from build123d import *

# Parameters (mm, degrees)
F1_DEPTH = 50.8
F2_DEPTH = 50.8
F3_DEPTH = 25.4
F4_DEPTH = 101.6
F5_SIZE  = 5
F6_R     = 5


with BuildPart() as f1:
    # F0 (on Front) → F1 (new body)
    with BuildSketch(Plane.XZ):
        with BuildLine():
            Line((-81.5396818683, 48.140194267), (-192.2345156552, 48.140194267))
            Line((-192.2345156552, 48.140194267), (-192.2345156552, 26.0968099283))
            ThreePointArc((-192.2345156552, 26.0968099283), (-174.3603015656, 18.6930680356), (-166.956559673, 0.8188539461))
            ThreePointArc((-166.956559673, 0.8188539461), (-174.3603015656, -17.0553601435), (-192.2345156552, -24.4591020361))
            Line((-192.2345156552, -24.4591020361), (-192.2345156552, -46.5024863749))
            Line((-192.2345156552, -46.5024863749), (-81.5396818683, -46.5024863749))
            ThreePointArc((-81.5396818683, -46.5024863749), (37.4445138693, -12.4899673839), (156.4287096069, -46.5024863749))
            Line((156.4287096069, -46.5024863749), (250.5448194923, -46.5024863749))
            Line((250.5448194923, -46.5024863749), (250.5448194923, -24.5132009882))
            ThreePointArc((250.5448194923, -24.5132009882), (225.212764558, 0.8188539461), (250.5448194923, 26.1509088804))
            Line((250.5448194923, 26.1509088804), (250.5448194923, 48.140194267))
            Line((250.5448194923, 48.140194267), (156.4287096069, 48.140194267))
            ThreePointArc((156.4287096069, 48.140194267), (37.4445138693, 1.7154132922), (-81.5396818683, 48.140194267))
        make_face()
    extrude(amount=F1_DEPTH)

    # F0 (on Front) → F2 (join)
    with BuildSketch(Plane.XZ):
        with BuildLine():
            Line((-81.5396818683, 48.140194267), (-192.2345156552, 48.140194267))
            Line((-192.2345156552, 48.140194267), (-192.2345156552, 26.0968099283))
            ThreePointArc((-192.2345156552, 26.0968099283), (-174.3603015656, 18.6930680356), (-166.956559673, 0.8188539461))
            ThreePointArc((-166.956559673, 0.8188539461), (-174.3603015656, -17.0553601435), (-192.2345156552, -24.4591020361))
            Line((-192.2345156552, -24.4591020361), (-192.2345156552, -46.5024863749))
            Line((-192.2345156552, -46.5024863749), (-81.5396818683, -46.5024863749))
            ThreePointArc((-81.5396818683, -46.5024863749), (37.4445138693, -12.4899673839), (156.4287096069, -46.5024863749))
            Line((156.4287096069, -46.5024863749), (250.5448194923, -46.5024863749))
            Line((250.5448194923, -46.5024863749), (250.5448194923, -24.5132009882))
            ThreePointArc((250.5448194923, -24.5132009882), (225.212764558, 0.8188539461), (250.5448194923, 26.1509088804))
            Line((250.5448194923, 26.1509088804), (250.5448194923, 48.140194267))
            Line((250.5448194923, 48.140194267), (156.4287096069, 48.140194267))
            ThreePointArc((156.4287096069, 48.140194267), (37.4445138693, 1.7154132922), (-81.5396818683, 48.140194267))
        make_face()
        with BuildLine():
            ThreePointArc((-166.956559673, 0.8188539461), (-174.3603015656, 18.6930680356), (-192.2345156552, 26.0968099283))
            Line((-192.2345156552, 26.0968099283), (-192.2345156552, 13.5188539461))
            ThreePointArc((-192.2345156552, 13.5188539461), (-183.2542595341, 9.7991100672), (-179.5345156552, 0.8188539461))
            ThreePointArc((-179.5345156552, 0.8188539461), (-183.2542595341, -8.161402175), (-192.2345156552, -11.8811460539))
            Line((-192.2345156552, -11.8811460539), (-192.2345156552, -24.4591020361))
            ThreePointArc((-192.2345156552, -24.4591020361), (-174.3603015656, -17.0553601435), (-166.956559673, 0.8188539461))
        make_face()
        with BuildLine():
            Line((-192.2345156552, 13.5188539461), (-192.2345156552, 26.0968099283))
            ThreePointArc((-192.2345156552, 26.0968099283), (-217.5124716374, 0.8188539461), (-192.2345156552, -24.4591020361))
            Line((-192.2345156552, -24.4591020361), (-192.2345156552, -11.8811460539))
            ThreePointArc((-192.2345156552, -11.8811460539), (-204.9345156552, 0.8188539461), (-192.2345156552, 13.5188539461))
        make_face()
        with BuildLine():
            ThreePointArc((275.8768744265, 0.8188539461), (268.4572873177, 18.7313217715), (250.5448194923, 26.1509088804))
            Line((250.5448194923, 26.1509088804), (250.5448194923, 13.5188539461))
            ThreePointArc((250.5448194923, 13.5188539461), (259.5250756133, 9.7991100672), (263.2448194923, 0.8188539461))
            ThreePointArc((263.2448194923, 0.8188539461), (259.5250756133, -8.161402175), (250.5448194923, -11.8811460539))
            Line((250.5448194923, -11.8811460539), (250.5448194923, -24.5132009882))
            ThreePointArc((250.5448194923, -24.5132009882), (268.4572873177, -17.0936138793), (275.8768744265, 0.8188539461))
        make_face()
        with BuildLine():
            Line((250.5448194923, 13.5188539461), (250.5448194923, 26.1509088804))
            ThreePointArc((250.5448194923, 26.1509088804), (225.212764558, 0.8188539461), (250.5448194923, -24.5132009882))
            Line((250.5448194923, -24.5132009882), (250.5448194923, -11.8811460539))
            ThreePointArc((250.5448194923, -11.8811460539), (237.8448194923, 0.8188539461), (250.5448194923, 13.5188539461))
        make_face()
    extrude(amount=F2_DEPTH)

    # F0 (on Front) → F3 (join)
    with BuildSketch(Plane.XZ):
        with BuildLine():
            Line((-81.5396818683, 48.140194267), (-192.2345156552, 48.140194267))
            Line((-192.2345156552, 48.140194267), (-192.2345156552, 26.0968099283))
            ThreePointArc((-192.2345156552, 26.0968099283), (-174.3603015656, 18.6930680356), (-166.956559673, 0.8188539461))
            ThreePointArc((-166.956559673, 0.8188539461), (-174.3603015656, -17.0553601435), (-192.2345156552, -24.4591020361))
            Line((-192.2345156552, -24.4591020361), (-192.2345156552, -46.5024863749))
            Line((-192.2345156552, -46.5024863749), (-81.5396818683, -46.5024863749))
            ThreePointArc((-81.5396818683, -46.5024863749), (37.4445138693, -12.4899673839), (156.4287096069, -46.5024863749))
            Line((156.4287096069, -46.5024863749), (250.5448194923, -46.5024863749))
            Line((250.5448194923, -46.5024863749), (250.5448194923, -24.5132009882))
            ThreePointArc((250.5448194923, -24.5132009882), (225.212764558, 0.8188539461), (250.5448194923, 26.1509088804))
            Line((250.5448194923, 26.1509088804), (250.5448194923, 48.140194267))
            Line((250.5448194923, 48.140194267), (156.4287096069, 48.140194267))
            ThreePointArc((156.4287096069, 48.140194267), (37.4445138693, 1.7154132922), (-81.5396818683, 48.140194267))
        make_face()
        with BuildLine():
            ThreePointArc((-166.956559673, 0.8188539461), (-174.3603015656, 18.6930680356), (-192.2345156552, 26.0968099283))
            Line((-192.2345156552, 26.0968099283), (-192.2345156552, 13.5188539461))
            ThreePointArc((-192.2345156552, 13.5188539461), (-183.2542595341, 9.7991100672), (-179.5345156552, 0.8188539461))
            ThreePointArc((-179.5345156552, 0.8188539461), (-183.2542595341, -8.161402175), (-192.2345156552, -11.8811460539))
            Line((-192.2345156552, -11.8811460539), (-192.2345156552, -24.4591020361))
            ThreePointArc((-192.2345156552, -24.4591020361), (-174.3603015656, -17.0553601435), (-166.956559673, 0.8188539461))
        make_face()
        with BuildLine():
            Line((-192.2345156552, 13.5188539461), (-192.2345156552, 26.0968099283))
            ThreePointArc((-192.2345156552, 26.0968099283), (-217.5124716374, 0.8188539461), (-192.2345156552, -24.4591020361))
            Line((-192.2345156552, -24.4591020361), (-192.2345156552, -11.8811460539))
            ThreePointArc((-192.2345156552, -11.8811460539), (-204.9345156552, 0.8188539461), (-192.2345156552, 13.5188539461))
        make_face()
        with BuildLine():
            ThreePointArc((275.8768744265, 0.8188539461), (268.4572873177, 18.7313217715), (250.5448194923, 26.1509088804))
            Line((250.5448194923, 26.1509088804), (250.5448194923, 13.5188539461))
            ThreePointArc((250.5448194923, 13.5188539461), (259.5250756133, 9.7991100672), (263.2448194923, 0.8188539461))
            ThreePointArc((263.2448194923, 0.8188539461), (259.5250756133, -8.161402175), (250.5448194923, -11.8811460539))
            Line((250.5448194923, -11.8811460539), (250.5448194923, -24.5132009882))
            ThreePointArc((250.5448194923, -24.5132009882), (268.4572873177, -17.0936138793), (275.8768744265, 0.8188539461))
        make_face()
        with BuildLine():
            Line((250.5448194923, 13.5188539461), (250.5448194923, 26.1509088804))
            ThreePointArc((250.5448194923, 26.1509088804), (225.212764558, 0.8188539461), (250.5448194923, -24.5132009882))
            Line((250.5448194923, -24.5132009882), (250.5448194923, -11.8811460539))
            ThreePointArc((250.5448194923, -11.8811460539), (237.8448194923, 0.8188539461), (250.5448194923, 13.5188539461))
        make_face()
    extrude(amount=F3_DEPTH)

    # F0 (on Front) → F4 (join)
    with BuildSketch(Plane.XZ):
        with BuildLine():
            ThreePointArc((-179.5345156552, 0.8188539461), (-183.2542595341, 9.7991100672), (-192.2345156552, 13.5188539461))
            ThreePointArc((-192.2345156552, 13.5188539461), (-204.9345156552, 0.8188539461), (-192.2345156552, -11.8811460539))
            ThreePointArc((-192.2345156552, -11.8811460539), (-183.2542595341, -8.161402175), (-179.5345156552, 0.8188539461))
        make_face()
    extrude(amount=F4_DEPTH)

    # F5
    f5_edges = [f1.edges().sort_by_distance(p)[0] for p in [
        (37.444514, 0, 1.715413),
        (37.444514, 0, -12.489967),
        (37.444514, -50.8, 1.715413),
        (37.444514, -50.8, -12.489967),
    ]]
    chamfer(f5_edges, length=F5_SIZE)

    # F6
    f6_edges = [f1.edges().sort_by_distance(p)[0] for p in [
        (-140.520101, 0, 48.140194),
        (-217.512472, 0, 0.818854),
        (-217.512472, -50.8, 0.818854),
    ]]
    fillet(f6_edges, radius=F6_R)


solid = f1.part
Here's how the part is built. I have some questions about the finished solid (model axes, mm). A direction names the side the tool comes from. Round coordinates to 2 decimals unless told otherwise and drop trailing zeros. Order: outer loops, then holes, each group sorted by start corner. A loop starts at its lowest first (then second) coordinate and runs counter-clockwise, first axis right, second up. Notation, with made-up numbers: M 64.5,77 L 117.5,77 A21 ccw 117.5,90 Z; hole C 21,62 d10. An arc over 180 degrees is marked long. Return JSON: item names as keys, results as strings. Group by question number.
1. If we section it at D-D on x = 190: List the corners of the cut face in (y, z) for me.
2. If we section it at A-A on y = -22: List the corners of the cut face in (x, z) for me.
3. Please list where these lines run through material, in increasing order: probe 1 along Y at (x, z) = (17, -2.5); probe 2 along X at (y, z) = (-26.5, -8); probe 3 along X at (y, z) = (-26, -4.5).
4. On a 3-axis mill with a long thin cutter (end or side, diameter ignored), from which of +Z, -Z, +X, -X, +Y, -Y can I reach the whole of each face in a straight line? I mean faces 5 (the face through (-217.506, -25.114, 1.375)), 6 (the face through (250.545, -25, 37)). Say none if no direction works.
5. I'm going to push flat-ended pins straight in: pin 1 Ø6.5 at (y, z) = (-36, -34) entering from +X; pin 2 Ø10 at (x, z) = (142, 9) entering from -Y; pin 3 Ø6 at (x, y) = (122, -42.5) entering from +Z; pin 4 Ø3 at (x, z) = (104.5, -6) entering from +Y. Where does each tip first touch, or does it pass through?
6. If we mould it in two halves opening along X, with no side actions, what happens to faces 1 (the face through (250.545, -25, -36)), 2 (the face through (-26, 0, 1)), 3 (the face through (39.274, -25.114, 1.725)), 4 (the face through (35.689, -25.114, -12.497))? For each: pulls with the +X half, pulls with the -X half, needs draft (parallel to the pull), parting line crosses it, or undercut.
7. If we section it at B-B on x = -156.5: List the corners of the cut face in (y, z) for me, then the cut area to 3 significant figures.
8. If we section it at C-C on y = -71.5: List the corners of the cut face in (x, z) for me.
Reply:
{
 "1": {"outline": "M -50.8,-46.5 L 0,-46.5 L 0,48.14 L -50.8,48.14 Z"},
 "2": {"outline": "M -192.23,-46.5 L -81.54,-46.5 A225.12 cw 156.43,-46.5 L 250.54,-46.5 L 250.54,-24.51 A25.33 ccw 250.54,26.15 L 250.54,48.14 L 156.43,48.14 A175.69 cw -81.54,48.14 L -192.23,48.14 L -192.23,26.1 A25.28 ccw -192.23,-24.46 Z; hole C 250.54,0.82 d25.4"},
 "3": {"probe 1": "-50.8 to 0", "probe 2": "-215.92 to 241.41, 259.68 to 274.29", "probe 3": "-216.95 to 239.01, 262.08 to 275.31"},
 "4": {"face 5": "-X, +Y, -Y", "face 6": "+Z, +X, +Y, -Y"},
 "5": {"pin 1": "x = 250.54", "pin 2": "y = -50.8", "pin 3": "z = 25.09", "pin 4": "y = 0"},
 "6": {"face 1": "pulls with the +X half", "face 2": "needs draft", "face 3": "undercut", "face 4": "undercut"},
 "7": {"outline": "M -50.8,-46.5 L 0,-46.5 L 0,43.14 A5 ccw -5,48.14 L -50.8,48.14 Z", "area": "4,800 mm^2"},
 "8": {"outline": "C -192.23,0.82 d25.4"}
}
